Model file for the job. Use its own axes, mm. A direction names the side the tool comes from. Round coordinates to 2 decimals unless told otherwise and drop trailing zeros. Loops run counter-clockwise (first coordinate to the right, second up) from the corner with the lowest first, then second, coordinate; pieces in that order, holes last.
from build123d import *

# Parameters (mm, degrees)
SKETCH_1_R                   = 1.7
EXTRUDE_1_DEPTH              = 6
EXTRUDE_3_DEPTH              = 14
FILLET_1_R                   = 1
FILLET_2_R                   = 10
HOLE_WIZARD_M3_1_D           = 3.4
HOLE_WIZARD_M3_1_DEPTH       = 20
HOLE_WIZARD_M3_1_CSINK_D     = 6.6
HOLE_WIZARD_M3_1_CSINK_ANGLE = 90
SKETCH_14_W                  = 15
SKETCH_14_H                  = 32
CUT_EXTRUDE_3_DEPTH          = 60.506302187
FILLET_3_R                   = 2


with BuildPart() as part:
    # 草图1 → 凸台-拉伸1 (new body)
    with BuildSketch(Plane(origin=(0, 0, 0), x_dir=(1, 0, 0), z_dir=(0, 1, 0))):
        with BuildLine():
            Line((-15.5, 3), (-15.5, -4))
            Line((-15.5, -4), (15.5, -4))
            Line((15.5, -4), (17.5, -4))
            Line((17.5, -4), (17.5, 8))
            ThreePointArc((17.5, 8), (17.124551632, 10.089119178), (16.045193687, 11.916786227))
            Line((16.045193687, 11.916786227), (-3.212338594, 34.263988522))
            ThreePointArc((-3.212338594, 34.263988522), (-8.449526575, 35.78527666), (-11.962215367, 31.613529665))
            Line((-11.962215367, 31.613529665), (-15.5, 3))
        make_face()
        with Locations(Location((-8, 0, 0), (0, 0, 270))):
            Circle(SKETCH_1_R, mode=Mode.SUBTRACT)
        with Locations(Location((-2.5, 8, 0), (0, 0, 270))):
            Circle(SKETCH_1_R, mode=Mode.SUBTRACT)
        with Locations(Location((8, 0, 0), (0, 0, 270))):
            Circle(SKETCH_1_R, mode=Mode.SUBTRACT)
        with Locations(Location((11.5, 8, 0), (0, 0, 270))):
            Circle(SKETCH_1_R, mode=Mode.SUBTRACT)
        with Locations(Location((-7, 31, 0), (0, 0, 270))):
            Circle(SKETCH_1_R, mode=Mode.SUBTRACT)
    extrude(amount=EXTRUDE_1_DEPTH)

    # 草图3 → 凸台-拉伸3 (add)
    with BuildSketch(Plane.XZ):
        Polygon((-15.120670115, -6.068012339), (-12.911963321, -23.931987661), (-8.911963321, -23.931987661), (-11.120670115, -6.068012339), align=None)
    extrude(amount=EXTRUDE_3_DEPTH)

    # 圆角1
    fillet_1_edges = [part.edges().sort_by_distance(p)[0] for p in [
        (17.5, 3, 4),
        (-15.5, 3, 4),
    ]]
    fillet(fillet_1_edges, radius=FILLET_1_R)

    # 圆角2
    fillet_2_edges = [part.edges().sort_by_distance(p)[0] for p in [
        (-15.5, 3, -3),
    ]]
    fillet(fillet_2_edges, radius=FILLET_2_R)

    # M3 十字槽半沉头木螺钉的锥形沉头孔1
    with Locations(Plane(origin=(0, 6, 0), x_dir=(1, 0, 0), z_dir=(0, 1, 0))):
        with Locations((-2.5, 8), (11.5, 8), (8, 0), (-8, 0), (-7, 31)):
            CounterSinkHole(HOLE_WIZARD_M3_1_D / 2, HOLE_WIZARD_M3_1_CSINK_D / 2, depth=HOLE_WIZARD_M3_1_DEPTH, counter_sink_angle=HOLE_WIZARD_M3_1_CSINK_ANGLE)

    # 镜向1: part across plane


with BuildPart() as part_1:
    add(part.part)
    add(part.part.mirror(Plane(origin=(0, -14, 0), x_dir=(0, 0, 1), z_dir=(0, -1, 0))))

    # 草图14 → 切除-拉伸3 (cut, through all)
    with BuildSketch(Plane(origin=(17.5, 0, 0), x_dir=(0, 0, -1), z_dir=(1, 0, 0))):
        with Locations((-4.4, -14)):
            Rectangle(SKETCH_14_W, SKETCH_14_H)
    extrude(amount=-CUT_EXTRUDE_3_DEPTH, mode=Mode.SUBTRACT)

    # 圆角3
    fillet_3_edges = [part_1.edges().sort_by_distance(p)[0] for p in [
        (-10.911963321, -28, -23.931987661),
        (-13.120670115, -28, -6.068012339),
        (-13.120670115, 0, -6.068012339),
        (-10.911963321, 0, -23.931987661),
    ]]
    fillet(fillet_3_edges, radius=FILLET_3_R)


solid = part_1.part
Q1. Slice it at C-C on z = 0. State how many separate pieces and enclosed holes the cut face has, plus the area to 3 significant figures.
Q2. Slice it at D-D on y = -5.5. Give the cut face in (x, z).
Q3. Tool access for faces 1 (the face through (-10.759, -27.43, -24.533)), 2 (the face through (1, 2, 0)), 3 (the face through (11.57, -30.17, -9.7)): list every direction of +Z, -Z, +X, -X, +Y, -Y with a clear straight run to the whole face (end or side of a thin tool).
Q4. Slice it at A-A on z = -31. Give the cut face in (x, y), plus the area to 3 significant figures.
Q5. Probe line 1 (X direction, y = 3.1, z = 0); line 2 (Y direction, x = -8, z = -5); line 3 (Y direction, x = 13, z = 0). List the from-to ranges inside material, lowest first.
Q6. Pull direction X, two halves, no side cores. Call faces 4 (the face through (-15.48, -31.71, -2.99)), 5 (the face through (-9.66, -31.18, -0.37)), 6 (the face through (-13.274, -0.601, -5.498)), 7 (the face through (-2.43, -30.17, -9.7)): pulls with the +X half, pulls with the -X half, needs draft (parallel to the pull), parting line crosses it, or undercut.
Q7. Slice it at B-B on x = -2.5. Give the cut face in (y, z), plus the area to 3 significant figures.
Q8. Flat gauge pins, fed straight in: P1, Ø5.5, axis at x = -7, z = -31, coming from the +Y side; P2, Ø2, axis at x = -7, z = -31, coming from the +Y side; P3, Ø3, axis at x = -13.5, y = -18, coming from the +Z side; P4, Ø8, axis at x = -5.5, z = 1.5, coming from the +Y side. Where does each tip first touch, or does it go through?
Reply:
1. separate pieces: 6
1. enclosed holes: 0
1. area: 199 mm2
2. outline: (-15.12, -6.07) - (-12.91, -23.93) - (-8.91, -23.93) - (-11.12, -6.07) - close
3. face 1: -Z, +X, -X
3. face 2: +Z, +X, -X
3. face 3: +Y, -Y
4. outline: (-12.04, -34) - (-10.3, -34) - (-8.7, -32.4) - (-8.7, -28) - (-12.04, -28) - close; (-12.04, 0) - (-8.7, 0) - (-8.7, 4.4) - (-10.3, 6) - (-12.04, 6) - close; (-5.3, -32.4) - (-3.7, -34) - (-0.4, -34) - (-0.4, -28) - (-5.3, -28) - close; (-5.3, 0) - (-0.4, 0) - (-0.4, 6) - (-3.7, 6) - (-5.3, 4.4) - close
4. area: 93.7 mm2
5. line 1: x = -15.5 to -9.7, -6.3 to 6.3, 9.7 to 17.5
5. line 2: y = -34 to -28, 0 to 6
5. line 3: y = -34 to -30, 2 to 6
6. face 4: pulls with the -X half
6. face 5: undercut
6. face 6: needs draft
6. face 7: undercut
7. outline: (-34, -33.44) - (-28, -33.44) - (-28, -9.7) - (-32.4, -9.7) - (-34, -11.3) - close; (-34, -4.7) - (-32.4, -6.3) - (-28, -6.3) - (-28, -3.1) - (-30, -3.1) - (-30, 4) - (-34, 4) - close; (0, -33.44) - (6, -33.44) - (6, -11.3) - (4.4, -9.7) - (0, -9.7) - close; (0, -6.3) - (4.4, -6.3) - (6, -4.7) - (6, 4) - (2, 4) - (2, -3.1) - (0, -3.1) - close
7. area: 375 mm2
8. P1: stops at y = 5.45
8. P2: passes through
8. P3: stops at z = -6.07
8. P4: stops at y = 6
